from build123d import *

# Parameters (mm, degrees)
SKETCH2_R           = 60
SKETCH2_R_2         = 5
BOSS_EXTRUDE1_DEPTH = 32
SKETCH4_R           = 5
CUT_EXTRUDE2_DEPTH  = 12
CUT_EXTRUDE3_DEPTH  = 12


with BuildPart() as part:
    # Sketch2 → Boss-Extrude1 (new body)
    with BuildSketch(Plane.XY):
        Circle(SKETCH2_R)
        Circle(SKETCH2_R_2, mode=Mode.SUBTRACT)
        with Locations((40, 0)):
            Circle(SKETCH2_R_2, mode=Mode.SUBTRACT)
        with Locations((-40, 0)):
            Circle(SKETCH2_R_2, mode=Mode.SUBTRACT)
        with Locations((0, 25)):
            Circle(SKETCH2_R_2, mode=Mode.SUBTRACT)
        with Locations((0, -25)):
            Circle(SKETCH2_R_2, mode=Mode.SUBTRACT)
    extrude(amount=BOSS_EXTRUDE1_DEPTH)

    # Sketch4 → Cut-Extrude2 (cut)
    with BuildSketch(Plane.XY):
        with BuildLine():
            Line((12, 12), (12, 25))
            ThreePointArc((12, 25), (0, 37), (-12, 25))
            Line((-12, 25), (-12, 12))
            Line((-12, 12), (-58.787753827, 12))
            ThreePointArc((-58.787753827, 12), (-60, 0), (-58.787753827, -12))
            Line((-58.787753827, -12), (-12, -12))
            Line((-12, -12), (-12, -25))
            ThreePointArc((-12, -25), (0, -37), (12, -25))
            Line((12, -25), (12, -12))
            Line((12, -12), (58.787753827, -12))
            ThreePointArc((58.787753827, -12), (59.69616918, -6.03053772), (60, 0))
            ThreePointArc((60, 0), (59.69616918, 6.03053772), (58.787753827, 12))
            Line((58.787753827, 12), (12, 12))
        make_face()
        with Locations((-40, 0)):
            Circle(SKETCH4_R, mode=Mode.SUBTRACT)
        with Locations((0, -25)):
            Circle(SKETCH4_R, mode=Mode.SUBTRACT)
        Circle(SKETCH4_R, mode=Mode.SUBTRACT)
        with Locations((40, 0)):
            Circle(SKETCH4_R, mode=Mode.SUBTRACT)
        with Locations((0, 25)):
            Circle(SKETCH4_R, mode=Mode.SUBTRACT)
    extrude(amount=CUT_EXTRUDE2_DEPTH, mode=Mode.SUBTRACT)

    # Sketch5 → Cut-Extrude3 (cut)
    with BuildSketch(Plane.XY):
        with BuildLine():
            ThreePointArc((27.613309165, 47.565798185), (0.130928127, 54.999844162), (-27.386534997, 47.696726312))
            ThreePointArc((-27.386534997, 47.696726312), (-29.602192231, 39.505825078), (-21.411290998, 37.290167844))
            ThreePointArc((-21.411290998, 37.290167844), (0.10236199, 42.999878163), (21.588587165, 37.187805854))
            ThreePointArc((21.588587165, 37.187805854), (29.789944331, 39.364441019), (27.613309165, 47.565798185))
        make_face()
        with BuildLine():
            ThreePointArc((-27.464289902, -47.832145212), (-29.679947137, -39.641243979), (-21.489045903, -37.425586744))
            ThreePointArc((-21.489045903, -37.425586744), (0.102733717, -43.156031824), (21.66698592, -37.322853027))
            ThreePointArc((21.66698592, -37.322853027), (29.868343086, -39.499488193), (27.69170792, -47.700845359))
            ThreePointArc((27.69170792, -47.700845359), (0.131299854, -55.155997823), (-27.464289902, -47.832145212))
        make_face()
    extrude(amount=CUT_EXTRUDE3_DEPTH, mode=Mode.SUBTRACT)


solid = part.part
Model file for the job. Use its own axes, mm. A direction names the side the tool comes from. Round coordinates to 2 decimals unless told otherwise and drop trailing zeros. Loops run counter-clockwise (first coordinate to the right, second up) from the corner with the lowest first, then second, coordinate; pieces in that order, holes last. Notation, with made-up numbers: (85.5, 34) -> (103.5, 34) arc R12 ccw to (103.5, 42) -> close; hole circle Ø5 at (33.5, -18.75). An arc over 180 degrees is marked (long way). Answer as CSV lines item,"result". Start each with the question number.
1) Slice it at A-A (x = 0). List the corners of the cut face in (y, z), plus the area to 3 significant figures.
2) Pin check, flat tips, straight feed: P1, Ø3.5, axis at x = -43.5, z = 5.5, coming from the +Y side; P2, Ø5, axis at x = 15, z = 15, coming from the +Y side; P3, Ø13, axis at y = 18, z = 4.5, coming from the -X side. Stop position of each tip, or through.
3) Slice it at D-D (z = 28). List the corners of the cut face in (x, y), plus the area to 3 significant figures.
4) Mould opens along X. For faces 4 (the face through (55.425, -22.98, 15.776)), 5 (the face through (0, 37, 6)), 6 (the face through (12, -30, 0)), 7 (the face through (-45, 0, 22)) say: +X half, -X half, draft (parallel to the pull), parting line (faces both ways), or undercut.
5) Probe line 1 along Y through (x, z) = (0, 23); line 2 along Y through (x, z) = (2, 29.5); line 3 along Z through (x, y) = (15, -8.5). List the from-to ranges inside material, lowest first.
6) Slice it at B-B (y = 0). List the corners of the cut face in (x, z), plus the area to 3 significant figures.
7) Tool access for faces 1 (the face through (-1.08, -4.88, 21.86)), 2 (the face through (36, 12, 6)), 3 (the face through (1, -46, 12)): list every direction of +Z, -Z, +X, -X, +Y, -Y with a clear straight run to the whole face (end or side of a thin tool).
8) Slice it at C-C (z = 7). List the corners of the cut face in (x, y).
Filled in:
1,outline,"(-60, 0) -> (-55.16, 0) -> (-55.16, 12) -> (-43.16, 12) -> (-43.16, 0) -> (-37, 0) -> (-37, 12) -> (-30, 12) -> (-30, 32) -> (-60, 32) -> close; (-20, 12) -> (-5, 12) -> (-5, 32) -> (-20, 32) -> close; (5, 12) -> (20, 12) -> (20, 32) -> (5, 32) -> close; (30, 12) -> (37, 12) -> (37, 0) -> (43, 0) -> (43, 12) -> (55, 12) -> (55, 0) -> (60, 0) -> (60, 32) -> (30, 32) -> close"
1,area,"2,060 mm2"
2,P1,"stops at y = 43.09"
2,P2,"stops at y = 58.68"
2,P3,"stops at x = -58.79"
3,outline,"circle Ø120 at (0, 0); hole circle Ø10 at (-40, 0); hole circle Ø10 at (0, -25); hole circle Ø10 at (0, 0); hole circle Ø10 at (0, 25); hole circle Ø10 at (40, 0)"
3,area,"10,900 mm2"
4,face 4,"parting line"
4,face 5,"undercut"
4,face 6,"draft"
4,face 7,"undercut"
5,line 1,"y = -60 to -30, -20 to -5, 5 to 20, 30 to 60"
5,line 2,"y = -59.97 to -29.58, -20.42 to -4.58, 4.58 to 20.42, 29.58 to 59.97"
5,line 3,"z = 12 to 32"
6,outline,"(-60, 12) -> (-45, 12) -> (-45, 32) -> (-60, 32) -> close; (-35, 12) -> (-5, 12) -> (-5, 32) -> (-35, 32) -> close; (5, 12) -> (35, 12) -> (35, 32) -> (5, 32) -> close; (45, 12) -> (60, 12) -> (60, 32) -> (45, 32) -> close"
6,area,"1,800 mm2"
7,face 1,"+Z, -Z"
7,face 2,"-Z, +X, -X"
7,face 3,"-Z"
8,outline,"(-58.79, -12) arc R60 ccw to (58.79, -12) -> (12, -12) -> (12, -25) arc R12 cw to (-12, -25) -> (-12, -12) -> close; (-58.79, 12) -> (-12, 12) -> (-12, 25) arc R12 cw to (12, 25) -> (12, 12) -> (58.79, 12) arc R60 ccw to start; hole (-27.46, -47.83) arc R55.16 ccw to (27.69, -47.7) arc R6 ccw to (21.67, -37.32) arc R43.16 cw to (-21.49, -37.43) arc R6 ccw to start; hole (-27.39, 47.7) arc R6 ccw to (-21.41, 37.29) arc R43 cw to (21.59, 37.19) arc R6 ccw to (27.61, 47.57) arc R55 ccw to start"
